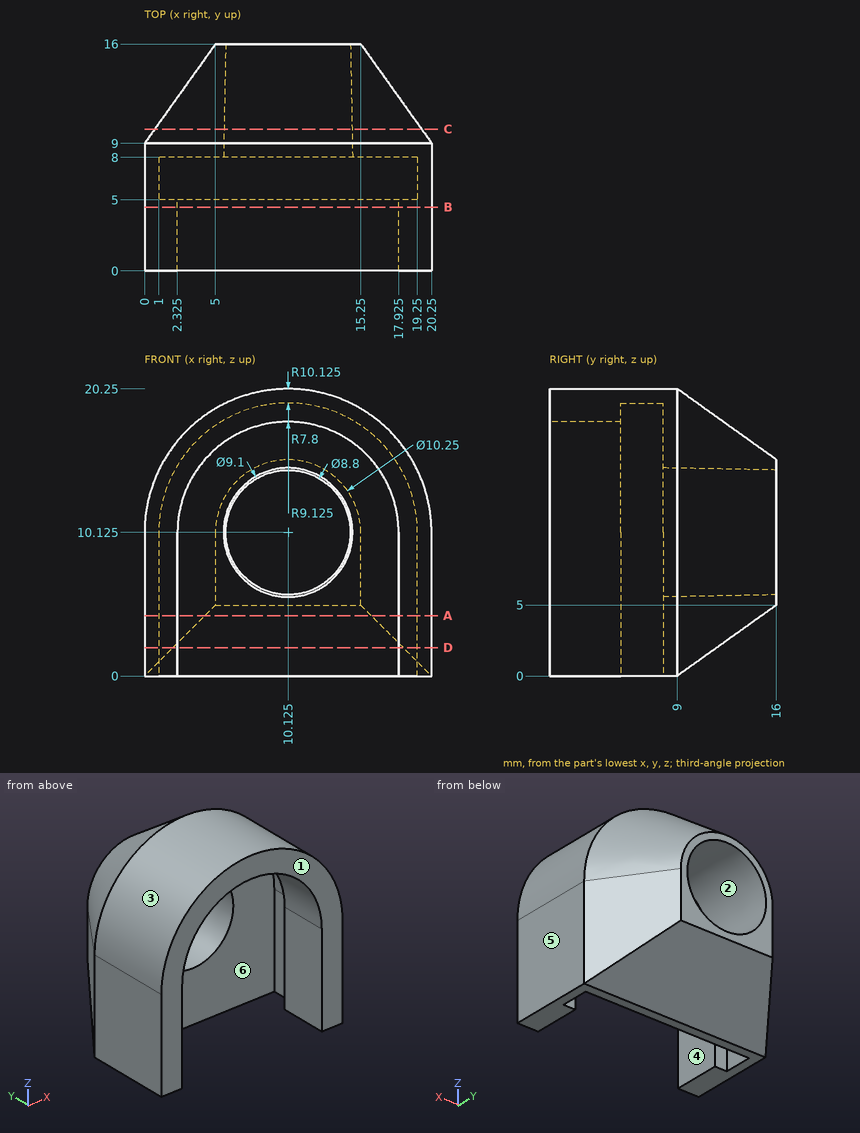
Geometry: see drawing. Coordinates: mm, zero at the bounding-box minimum. A direction names the side the tool comes from. Give positions to 0.01 mm unless a question says otherwise; leave off trailing zeros. Loops run counter-clockwise (first coordinate to the right, second up) from the corner with the lowest first, then second, coordinate; pieces in that order, holes last. Notation, with made-up numbers: (42, 37.5) -> (97, 37.5) arc R14 ccw to (97, 49.5) -> close; hole circle Ø11 at (-19.5, 25). An arc over 180 degrees is marked (long way). Use CSV: the item, a comma, the result in double quotes.
(1) Access query for the marked faces 4, 5 and 6. Directions: +Z, -Z, +X, -X, +Y, -Y. A direction counts if a zero-diameter tool reaches every point of the face in a straight line with its end or side. Return the directions, or none.
From the geometry:
face 4,"-Z, -Y"
face 5,"+Z, -Z, +X, +Y, -Y"
face 6,"-Z"
(2) Cut plane A-A (z = 4.25). Output: boundary loops of the cut face in (x, y) (3 decimals).
From the geometry:
outline,"(0, 0) -> (2.325, 0) -> (2.325, 5) -> (1, 5) -> (1, 8) -> (19.25, 8) -> (19.25, 5) -> (17.925, 5) -> (17.925, 0) -> (20.25, 0) -> (20.25, 9) -> (16, 14.95) -> (4.25, 14.95) -> (0, 9) -> close"
(3) First-contact query: P1, Ø6, axis at x = 6, z = 3.5, coming from the -Y side; P2, Ø6, axis at y = 13.5, z = 11.5, coming from the +X side; P3, Ø8, axis at x = 2, y = 13.5, coming from the -Z side. Flat tips, straight axial feed; report the tip coordinate or a pass-through.
From the geometry:
P1,"y = 8"
P2,"x = 19.11"
P3,"z = 0.36"
(4) Cut plane B-B (y = 4.5). Output: boundary loops of the cut face in (x, z) (3 decimals), plus the area to 3 significant figures.
From the geometry:
outline,"(0, 0) -> (2.325, 0) -> (2.325, 10.125) arc R7.8 cw to (17.925, 10.125) -> (17.925, 0) -> (20.25, 0) -> (20.25, 10.125) arc R10.125 ccw to (0, 10.125) -> close"
area,"113 mm^2"
(5) Ray query, line 1 along X through (y, z) = (7.25, 4); line 2 along X through (y, z) = (1.5, 1.25) (3 decimals); line 3 along Y through (x, z) = (8, 14.25). Return the intervals inside material, ascending. Write a range as [from, to].
From the geometry:
line 1,"[0, 1], [19.25, 20.25]"
line 2,"[0, 2.325], [17.925, 20.25]"
line 3,"[8, 16]"
(6) Cut plane C-C (y = 10). Output: boundary loops of the cut face in (x, z) (1 decimal), plus the area to 3 significant figures.
From the geometry:
outline,"(0.7, 0.7) -> (19.5, 0.7) -> (19.5, 10.1) arc R9.4 ccw to (0.7, 10.1) -> close; hole circle Ø9 at (10.1, 10.1)"
area,"252 mm^2"
(7) Pull-direction query (X, two-part tool) for the marked faces 1, 2 and 3; classes: released by +X, released by -X, zero draft, split by the parting line, or undercut.
From the geometry:
face 1,"zero draft"
face 2,"undercut"
face 3,"split by the parting line"
(8) Cut plane D-D (z = 2). Output: boundary loops of the cut face in (x, y) (3 decimals), plus the area to 3 significant figures.
From the geometry:
outline,"(0, 0) -> (2.325, 0) -> (2.325, 5) -> (1, 5) -> (1, 8) -> (19.25, 8) -> (19.25, 5) -> (17.925, 5) -> (17.925, 0) -> (20.25, 0) -> (20.25, 9) -> (18.25, 11.8) -> (2, 11.8) -> (0, 9) -> close"
area,"101 mm^2"
